Work out the finished part from the listing and answer in its coordinate system (mm). Give positions to 0.01 mm unless a question says otherwise; leave off trailing zeros. Loops run counter-clockwise (first coordinate to the right, second up) from the corner with the lowest first, then second, coordinate; pieces in that order, holes last.
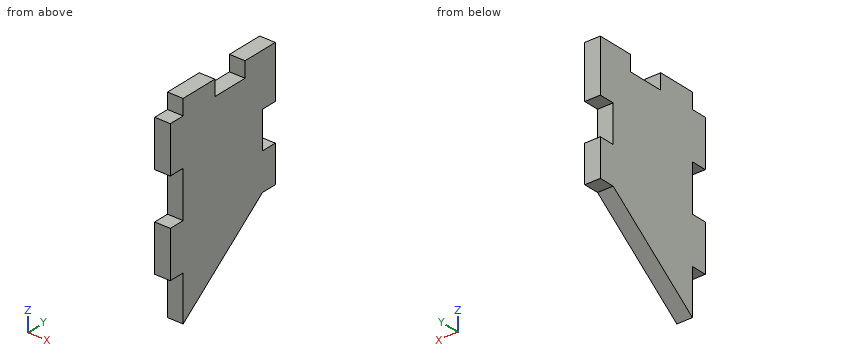
```python
from build123d import *

# Parameters (mm, degrees)
SKETCH1_W            = 63.5
SKETCH1_H            = 33.02
BOSS_EXTRUDE1_DEPTH  = 5.334
CUT_EXTRUDE1_DEPTH   = 6.334
SKETCH3_W            = 12.7
SKETCH3_H            = 5.334
SKETCH3_W_2          = 15.971321783
BOSS_EXTRUDE2_DEPTH  = 5.334
SKETCH4_W            = 5.334
SKETCH4_H            = 37.084
BOSS_EXTRUDE7_DEPTH  = 5.334
SKETCH5_W            = 5.334
SKETCH5_H            = 12.573
CUT_EXTRUDE2_DEPTH   = 6.334
SKETCH6_W            = 5.334
SKETCH6_H            = 0.635
BOSS_EXTRUDE9_DEPTH  = 5.334
SKETCH7_W            = 5.334
SKETCH7_H            = 0.635
BOSS_EXTRUDE10_DEPTH = 5.334


with BuildPart() as part:
    # Sketch1 → Boss-Extrude1 (new body)
    with BuildSketch(Plane(origin=(0, 0, 0), x_dir=(0, 0, -1), z_dir=(1, 0, 0))):
        Rectangle(SKETCH1_W, SKETCH1_H)
    extrude(amount=BOSS_EXTRUDE1_DEPTH)

    # Sketch2 → Cut-Extrude1 (cut, through all)
    with BuildSketch(Plane.ZY):
        Polygon((-31.75, -16.51), (-31.75, 16.51), (-6.35, 16.51), align=None)
    extrude(amount=-CUT_EXTRUDE1_DEPTH, mode=Mode.SUBTRACT)

    # Sketch3 → Boss-Extrude2 (add, through all)
    with BuildSketch(Plane.ZY):
        with Locations((25.4, 19.177)):
            Rectangle(SKETCH3_W, SKETCH3_H)
        with Locations((0, 19.177)):
            Rectangle(SKETCH3_W, SKETCH3_H)
        with Locations((23.764339109, -19.177)):
            Rectangle(SKETCH3_W_2, SKETCH3_H)
        with Locations((-8.178304458, -19.177)):
            Rectangle(SKETCH3_W_2, SKETCH3_H)
    extrude(amount=-BOSS_EXTRUDE2_DEPTH)

    # Sketch4 → Boss-Extrude7 (add)
    with BuildSketch(Plane.ZY):
        with Locations((34.417, 2.667)):
            Rectangle(SKETCH4_W, SKETCH4_H)
    extrude(amount=-BOSS_EXTRUDE7_DEPTH)

    # Sketch5 → Cut-Extrude2 (cut, through all)
    with BuildSketch(Plane(origin=(5.334, 0, 0), x_dir=(0, 0, -1), z_dir=(1, 0, 0))):
        with Locations((-34.417, 2.9845)):
            Rectangle(SKETCH5_W, SKETCH5_H)
    extrude(amount=-CUT_EXTRUDE2_DEPTH, mode=Mode.SUBTRACT)

    # Sketch6 → Boss-Extrude9 (add)
    with BuildSketch(Plane(origin=(5.334, 0, 0), x_dir=(0, 0, -1), z_dir=(1, 0, 0))):
        with Locations((-34.417, 21.5265)):
            Rectangle(SKETCH6_W, SKETCH6_H)
    extrude(amount=-BOSS_EXTRUDE9_DEPTH)

    # Sketch7 → Boss-Extrude10 (add)
    with BuildSketch(Plane(origin=(5.334, 0, 0), x_dir=(0, 0, -1), z_dir=(1, 0, 0))):
        with Locations((-34.417, -16.1925)):
            Rectangle(SKETCH7_W, SKETCH7_H)
    extrude(amount=-BOSS_EXTRUDE10_DEPTH)


solid = part.part
```
Q1. Section A-A on x = 3.9 is taken. Give the vertices of the cut face in (y, z), plus the area to 3 significant figures.
Q2. Consider line 1 along Y through (x, z) = (1, 5); line 2 along Y through (x, z) = (2.2, 13.5); line 3 along Z through (x, y) = (2.5, -20). Determine where each line is inside the solid, lowest interval first.
Q3. Section B-B on z = 11 is taken. Give the vertices of the cut face in (x, y).
Q4. Given pin 1 (2.5 mm diameter, centred on x = 1.5, y = 19.5, fed in from -Z); pin 2 (2.5 mm diameter, centred on x = 3.5, y = -18.5, fed in from +Z); pin 3 (1.6 mm diameter, centred on x = 4, z = 34, fed in from -Y), each flat-ended and moving along its own axis, determine where each tip first touches the part or whether it passes through.
Q5. Section C-C on y = 14.5 is taken. Give the vertices of the cut face in (x, z).
Check result:
1. outline: (-21.84, -16.16) - (-16.51, -16.16) - (-16.51, -31.75) - (16.51, -6.35) - (21.84, -6.35) - (21.84, 6.35) - (16.51, 6.35) - (16.51, 19.05) - (21.84, 19.05) - (21.84, 37.08) - (9.27, 37.08) - (9.27, 31.75) - (-3.3, 31.75) - (-3.3, 37.08) - (-16.51, 37.08) - (-16.51, 31.75) - (-21.84, 31.75) - (-21.84, 15.78) - (-16.51, 15.78) - (-16.51, -0.19) - (-21.84, -0.19) - close
1. area: 2,120 mm2
2. line 1: y = -16.51 to 21.84
2. line 2: y = -16.51 to 16.51
2. line 3: z = -16.16 to -0.19, 15.78 to 31.75
3. outline: (0, -16.51) - (5.33, -16.51) - (5.33, 16.51) - (0, 16.51) - close
4. pin 1: stops at z = -6.35
4. pin 2: stops at z = 31.75
4. pin 3: stops at y = -16.51
5. outline: (0, -7.9) - (5.33, -7.9) - (5.33, 37.08) - (0, 37.08) - close
